Can you work these out from the model? Positions are in its coordinate system, mm. Face numbers are marked on the shaded views. A direction names the side the tool comes from. Give positions to 0.01 mm unless a question says otherwise; leave off trailing zeros. Loops run counter-clockwise (first coordinate to the right, second up) from the corner with the lowest first, then second, coordinate; pieces in that order, holes last. Notation, with made-up numbers: (-5, -5) - (31, -5) arc R23 ccw to (31, 20) - close; hole circle Ø7 at (-24.5, 53.5). An arc over 180 degrees is marked (long way). Answer in a Markdown table with one row per item.
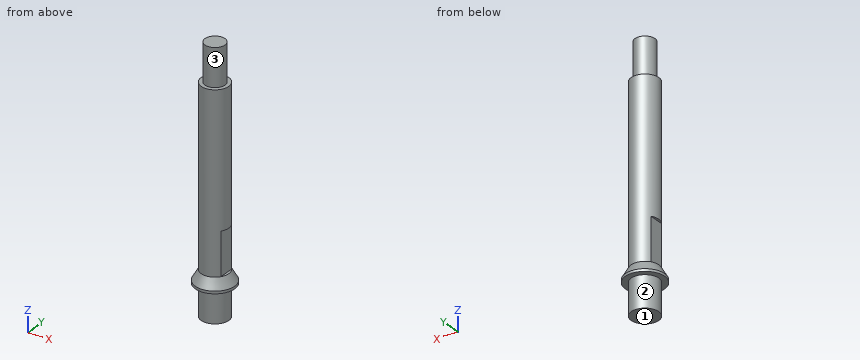
from build123d import *

# Parameters (mm, degrees)
SKETCH1_R           = 11
BOSS_EXTRUDE1_DEPTH = 140
SKETCH2_R           = 8
BOSS_EXTRUDE2_DEPTH = 30
SKETCH3_R           = 11
BOSS_EXTRUDE3_DEPTH = 8
BOSS_EXTRUDE3_DRAFT = -30
SKETCH4_R           = 15.618802154
BOSS_EXTRUDE4_DEPTH = 2
SKETCH5_W           = 34.053216137
SKETCH5_H           = 15
CUT_EXTRUDE1_DEPTH  = 2
BOSS_EXTRUDE5_START = 25
SKETCH6_R           = 11
BOSS_EXTRUDE5_DEPTH = 25


with BuildPart() as part:
    # Sketch1 → Boss-Extrude1 (new body)
    with BuildSketch(Plane.XY):
        Circle(SKETCH1_R)
    extrude(amount=BOSS_EXTRUDE1_DEPTH)

    # Sketch2 → Boss-Extrude2 (add)
    with BuildSketch(Plane.XY.offset(140)):
        Circle(SKETCH2_R)
    extrude(amount=BOSS_EXTRUDE2_DEPTH)


with BuildPart() as boss_extrude3_tool:
    # Sketch3 → Boss-Extrude3 (with draft: the straight prism first)
    with BuildSketch(Plane(origin=(0, 0, 0), x_dir=(-1, 0, 0), z_dir=(0, 0, -1))):
        Circle(SKETCH3_R)
    extrude(amount=BOSS_EXTRUDE3_DEPTH)
    # Boss-Extrude3: the draft: its side faces are tilted about the plane it starts from
    boss_extrude3_sides = [boss_extrude3_tool.faces().sort_by_distance(p)[0] for p in [
        (11, 0, -4),
    ]]
    draft(boss_extrude3_sides, Plane(origin=(0, 0, 0), x_dir=(-1, 0, 0), z_dir=(0, 0, -1)), BOSS_EXTRUDE3_DRAFT)


with BuildPart() as part_1:
    add(part.part)

    # Boss-Extrude3: add boss_extrude3_tool
    add(boss_extrude3_tool.part)

    # Sketch4 → Boss-Extrude4 (add)
    with BuildSketch(Plane(origin=(0, 0, -8), x_dir=(-1, 0, 0), z_dir=(0, 0, -1))):
        Circle(SKETCH4_R)
    extrude(amount=BOSS_EXTRUDE4_DEPTH)

    # Sketch5 → Cut-Extrude1 (cut)
    with BuildSketch(Plane.ZY.offset(11)):
        with Locations((17.026608068, 0)):
            Rectangle(SKETCH5_W, SKETCH5_H)
    cut_extrude1 = extrude(amount=-CUT_EXTRUDE1_DEPTH, mode=Mode.SUBTRACT)

    # Mirror1: Cut-Extrude1 across plane
    add(cut_extrude1.mirror(Plane(origin=(0, 0, 0), x_dir=(0, 0, 1), z_dir=(1, 0, 0))), mode=Mode.SUBTRACT)

    # Sketch6 → Boss-Extrude5 (add)
    with BuildSketch(Plane(origin=(0, 0, -10), x_dir=(-1, 0, 0), z_dir=(0, 0, -1)).offset(BOSS_EXTRUDE5_START)):
        with Locations(Location((0, 0, 0), (0, 0, 35.096801228))):
            Circle(SKETCH6_R)
    extrude(amount=-BOSS_EXTRUDE5_DEPTH)


solid = part_1.part
Q1. Imagine slicing it at B-B, the plane x = 0. Write out the boundary of the cut face in (y, z).
Checked values:
| item | result |
|---|---|
| outline | (-15.62, -10) - (-11, -10) - (-11, -35) - (11, -35) - (11, -10) - (15.62, -10) - (15.62, -8) - (11, 0) - (11, 140) - (8, 140) - (8, 170) - (-8, 170) - (-8, 140) - (-11, 140) - (-11, 0) - (-15.62, -8) - close |
Q2. On a 3-axis mill with a long thin cutter (end or side, diameter ignored), from which of +Z, -Z, +X, -X, +Y, -Y can I reach the whole of each face in a straight line? I mean the marked faces 1, 2 and 3. Say none if no direction works.
Checked values:
| item | result |
|---|---|
| face 1 | -Z, +X, -X, +Y, -Y |
| face 2 | -Z |
| face 3 | +Z |
Q3. If I drill on line 1 (Z direction, x = 7.5, y = -4.5); line 2 (Y direction, x = -0.5, z = 114.5); line 3 (X direction, y = -2, z = 9.5), over which ranges is the centre line in solid material (lowest first)? Write a range as [from, to].
Checked values:
| item | result |
|---|---|
| line 1 | z = [-35, 140] |
| line 2 | y = [-10.99, 10.99] |
| line 3 | x = [-9, 9] |
Q4. For pin 1 (2 mm diameter, centred on x = 10.5, z = 18, fed in from -Y); pin 2 (3 mm diameter, centred on x = 12.5, y = 6.5, fed in from -Z); pin 3 (1 mm diameter, centred on x = -10, y = -2, fed in from +Z); pin 4 (10 mm diameter, centred on x = 2, z = 148.5, fed in from -Y), each with a flat end and sliding along its axis, tell me the tip position at first contact or that it passes through.
Checked values:
| item | result |
|---|---|
| pin 1 | passes through |
| pin 2 | stops at z = -10 |
| pin 3 | stops at z = 140 |
| pin 4 | stops at y = -8 |
Q5. Imagine slicing it at D-D, the plane z = 134. Write out the boundary of the cut face in (x, y), and give its area (3 significant figures).
Checked values:
| item | result |
|---|---|
| outline | circle Ø22 at (0, 0) |
| area | 380 mm² |
Q6. Imagine slicing it at C-C, the plane z = 5.5. Write out the boundary of the cut face in (x, y).
Checked values:
| item | result |
|---|---|
| outline | (-9, -6.32) arc R11 ccw to (9, -6.32) - (9, 6.32) arc R11 ccw to (-9, 6.32) - close |
Q7. Imagine slicing it at A-A, the plane y = 0. Write out the boundary of the cut face in (x, z), and give its area (3 significant figures).
Checked values:
| item | result |
|---|---|
| outline | (-15.62, -10) - (-11, -10) - (-11, -35) - (11, -35) - (11, -10) - (15.62, -10) - (15.62, -8) - (11, 0) - (9, 0) - (9, 34.05) - (11, 34.05) - (11, 140) - (8, 140) - (8, 170) - (-8, 170) - (-8, 140) - (-11, 140) - (-11, 34.05) - (-9, 34.05) - (-9, 0) - (-11, 0) - (-15.62, -8) - close |
| area | 4,250 mm² |
